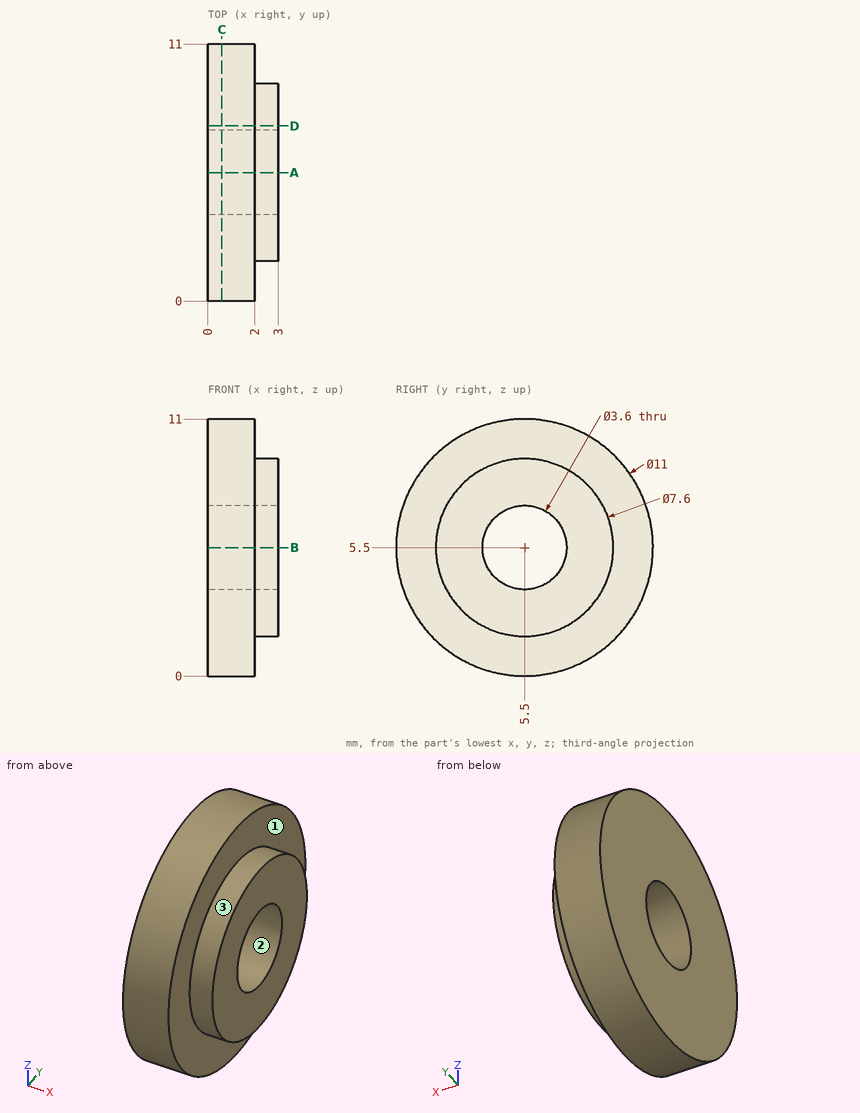
Input: dimensioned drawing with shaded views. Units: mm. Origin: part minimum x, y, z. Round coordinates to 2 decimals unless told otherwise and drop trailing zeros. Loops run counter-clockwise (first coordinate to the right, second up) from the corner with the lowest first, then second, coordinate; pieces in that order, holes last. Notation, with made-up numbers: (-38, 12.5) -> (-8, 12.5) arc R16 cw to (-8, 19.5) -> close; hole circle Ø10 at (-28.75, 30.5). An arc over 180 degrees is marked (long way). Use one line per item in the form item = value. Start each with the question number.
1) Section C-C on x = 0.6. Output: boundary loops of the cut face in (y, z), then the cut area to 3 significant figures.
2) First-contact query: P1, Ø1.5, axis at x = 2.5, y = 6, coming from the +Z side. Flat tip, straight axial feed; report the tip coordinate or a pass-through.
3) Line query: L1, parallel to Y at x = 1.7, z = 5.5; L2, parallel to X at y = 1, z = 2.5; L3, parallel to Z at x = 1.8, y = 5.25. Output: solid intervals per line, ascending.
4) Draft query along Z for the marked faces 1, 2 and 3. Return one class per face: released by +Z, released by -Z, zero draft, split by the parting line, or undercut.
5) Section D-D on y = 7.5. Output: boundary loops of the cut face in (x, z), then the cut area to 3 significant figures.
6) Section A-A on y = 5.5. Output: boundary loops of the cut face in (x, z), then the cut area to 3 significant figures.
Response:
q1.outline = circle Ø11 at (5.5, 5.5); hole circle Ø3.6 at (5.5, 5.5)
q1.area = 84.9 mm^2
q2.P1 = 11
q3.L1 = 0 to 3.7, 7.3 to 11
q3.L2 = 0 to 2
q3.L3 = 0.01 to 3.72, 7.28 to 10.99
q4.face_1 = zero draft
q4.face_2 = undercut
q4.face_3 = split by the parting line
q5.outline = (0, 0.38) -> (2, 0.38) -> (2, 2.27) -> (3, 2.27) -> (3, 8.73) -> (2, 8.73) -> (2, 10.62) -> (0, 10.62) -> close
q5.area = 27.0 mm^2
q6.outline = (0, 0) -> (2, 0) -> (2, 1.7) -> (3, 1.7) -> (3, 3.7) -> (0, 3.7) -> close; (0, 7.3) -> (3, 7.3) -> (3, 9.3) -> (2, 9.3) -> (2, 11) -> (0, 11) -> close
q6.area = 18.8 mm^2
